Here's how the part is built. I have some questions about the finished solid (model axes, mm). A direction names the side the tool comes from. Coordinates: 2 decimals unless noted, no trailing zeros. Loops run counter-clockwise (first coordinate to the right, second up) from the corner with the lowest first, then second, coordinate; pieces in that order, holes last. Notation, with made-up numbers: (-38, 86) -> (-28, 86) arc R7 ccw to (-28, 90) -> close; hole circle Ø6 at (26, 54). An arc over 180 degrees is marked (long way). Answer as a JSON object with one key per item and string values. Group by question number.
Q1. Thinking about a two-plate mould opening in Y: for faces 1 (the flat face through (12.7, -4.3, 0.1)), 2 (the cylindrical face through (7.28, -9.76, 2.17)), 3 (the flat face through (6, 5.422, 0)), which applies, released by +Y, released by -Y, zero draft, split by the parting line, or undercut?
Q2. I want a section at A-A on y = 0. Write out the boundary of the cut face in (x, z), then the cut area to 3 significant figures.
Q3. I want a section at D-D on y = -8. Write out the boundary of the cut face in (x, z).
Q4. I want a section at C-C on x = 2.5. Write out the boundary of the cut face in (y, z).
Q5. I want a section at B-B on z = 0. Write out the boundary of the cut face in (x, y), then the cut area to 3 significant figures.
Q6. I need wall thicknesses on line 1 (Y direction, x = 3, z = 0); line 2 (Z direction, x = 4.5, y = 0); line 3 (Y direction, x = 11.5, z = 3.5). Which ranges of each line are inside material? Lowest first, please.
Q7. I'm going to push flat-ended pins straight in: pin 1 (1.5 mm diameter, centred on x = 5, z = -0.5, fed in from -Y); pin 2 (6 mm diameter, centred on x = 6, y = 1.5, fed in from -Z); pin 3 (0.7 mm diameter, centred on x = 7, y = 4.5, fed in from -Z). Where does each tip first touch, or does it pass through?
Q8. On a 3-axis mill with a long thin cutter (end or side, diameter ignored), from which of +Z, -Z, +X, -X, +Y, -Y can I reach the whole of each face in a straight line? I mean faces 4 (the flat face through (6, 4, -2.5)), 5 (the flat face through (2, 5, -9)), 6 (the flat face through (0, -5, 0)). Say none if no direction works.
```python
from build123d import *

# Parameters (mm, degrees)
SKETCH1_R           = 10
BOSS_EXTRUDE1_DEPTH = 12.7
SKETCH2_R           = 11.5
SKETCH2_R_2         = 10
BOSS_EXTRUDE2_DEPTH = 2


with BuildPart() as part:
    # Sketch1 → Boss-Extrude1 (new body)
    with BuildSketch(Plane(origin=(0, 0, 0), x_dir=(0, 0, -1), z_dir=(1, 0, 0))):
        Circle(SKETCH1_R)
        with BuildLine():
            Line((-2.5, 5.422498999), (2.5, 5.422498999))
            Line((2.5, 5.422498999), (2.5, 3.122498999))
            ThreePointArc((2.5, 3.122498999), (0, -4), (-2.5, 3.122498999))
            Line((-2.5, 3.122498999), (-2.5, 5.422498999))
        make_face(mode=Mode.SUBTRACT)
    extrude(amount=BOSS_EXTRUDE1_DEPTH)

    # Sketch2 → Boss-Extrude2 (add)
    with BuildSketch(Plane.ZY):
        Circle(SKETCH2_R)
        Circle(SKETCH2_R_2, mode=Mode.SUBTRACT)
    extrude(amount=-BOSS_EXTRUDE2_DEPTH)


solid = part.part
```
Result set:
{
 "1": {"face 1": "zero draft", "face 2": "split by the parting line", "face 3": "undercut"},
 "2": {"outline": "(0, -11.5) -> (2, -11.5) -> (2, -10) -> (12.7, -10) -> (12.7, -4) -> (0, -4) -> close; (0, 4) -> (12.7, 4) -> (12.7, 10) -> (2, 10) -> (2, 11.5) -> (0, 11.5) -> close", "area": "158 mm²"},
 "3": {"outline": "(0, -8.26) -> (2, -8.26) -> (2, -6) -> (12.7, -6) -> (12.7, 6) -> (2, 6) -> (2, 8.26) -> (0, 8.26) -> close"},
 "4": {"outline": "circle Ø20 at (0, 0); hole (3.12, -2.5) -> (5.42, -2.5) -> (5.42, 2.5) -> (3.12, 2.5) arc R4 ccw (long way) to start"},
 "5": {"outline": "(0, -11.5) -> (2, -11.5) -> (2, -10) -> (12.7, -10) -> (12.7, -4) -> (0, -4) -> close; (0, 5.42) -> (12.7, 5.42) -> (12.7, 10) -> (2, 10) -> (2, 11.5) -> (0, 11.5) -> close", "area": "140 mm²"},
 "6": {"line 1": "y = -10 to -4, 5.42 to 10", "line 2": "z = -10 to -4, 4 to 10", "line 3": "y = -9.37 to -1.94, 1.94 to 9.37"},
 "7": {"pin 1": "stops at y = -10", "pin 2": "stops at z = -10", "pin 3": "stops at z = -9.1"},
 "8": {"face 4": "+X, -X", "face 5": "+X", "face 6": "+Z, -Z, -X, +Y, -Y"}
}
